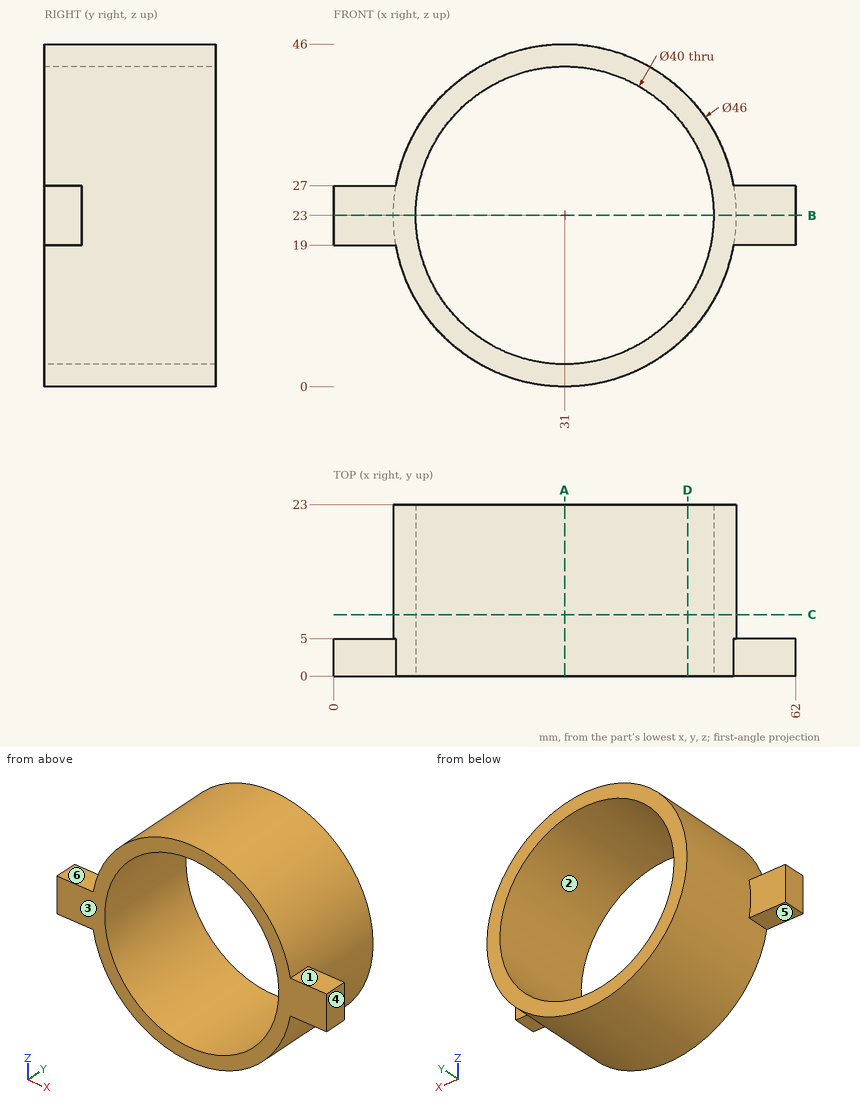
Job drawing, mm, ordinate dimensions from the low corner. One solid piece. A direction names the side the tool comes from. Give positions to 0.01 mm unless a question says otherwise; leave off trailing zeros. Loops run counter-clockwise (first coordinate to the right, second up) from the corner with the lowest first, then second, coordinate; pieces in that order, holes last. Notation, with made-up numbers: (81.25, 24.25) -> (138.25, 24.25) arc R13 ccw to (138.25, 39.25) -> close; hole circle Ø11 at (-16.75, -20.5). An arc over 180 degrees is marked (long way). Use a Markdown table: item, result. Add a question column.
(1) Slice it at C-C on y = 8.25. List the corners of the cut face in (x, z), and give its area (3 significant figures).
(2) Mould opens along Z. For the marked faces 1, 2 and 3 say: +Z half, -Z half, draft (parallel to the pull), parting line (faces both ways), or undercut.
(3) Slice it at B-B on z = 23. List the corners of the cut face in (x, y).
(4) Wall check: line 1 along X through (y, z) = (17, 23); line 2 along Y through (x, z) = (6, 20); line 3 along Z through (x, y) = (46, 14). Give the ranges that are in metal, low to high.
(5) Slice it at D-D on x = 47.5. List the corners of the cut face in (y, z), and give its area (3 significant figures).
(6) Tool access for the marked faces 4, 5 and 6: list every direction of +Z, -Z, +X, -X, +Y, -Y with a clear straight run to the whole face (end or side of a thin tool).
(7) Slice it at A-A on x = 31. List the corners of the cut face in (y, z), and give its area (3 significant figures).
(8) Drop flat-ended pins along their axis: pin 1 Ø4 at (y, z) = (20, 38) entering from -X; pin 2 Ø9 at (x, z) = (59, 24) entering from +Y; pin 3 Ø1.5 at (x, y) = (15, 6.5) entering from +Z. Give the stop position or say it passes through.
Filled sheet:
| question | item | result |
|---|---|---|
| 1 | outline | circle Ø46 at (31, 23); hole circle Ø40 at (31, 23) |
| 1 | area | 405 mm2 |
| 2 | face 1 | +Z half |
| 2 | face 2 | undercut |
| 2 | face 3 | draft |
| 3 | outline | (0, 0) -> (11, 0) -> (11, 23) -> (8, 23) -> (8, 5) -> (0, 5) -> close; (51, 0) -> (62, 0) -> (62, 5) -> (54, 5) -> (54, 23) -> (51, 23) -> close |
| 4 | line 1 | 8 to 11, 51 to 54 |
| 4 | line 2 | 0 to 5 |
| 4 | line 3 | 5.56 to 9.77, 36.23 to 40.44 |
| 5 | outline | (0, 6.98) -> (23, 6.98) -> (23, 11.7) -> (0, 11.7) -> close; (0, 34.3) -> (23, 34.3) -> (23, 39.02) -> (0, 39.02) -> close |
| 5 | area | 217 mm2 |
| 6 | face 4 | +Z, -Z, +X, +Y, -Y |
| 6 | face 5 | -Z, -X, +Y, -Y |
| 6 | face 6 | +Z, -X, +Y, -Y |
| 7 | outline | (0, 0) -> (23, 0) -> (23, 3) -> (0, 3) -> close; (0, 43) -> (23, 43) -> (23, 46) -> (0, 46) -> close |
| 7 | area | 138 mm2 |
| 8 | pin 1 | x = 12.03 |
| 8 | pin 2 | y = 5 |
| 8 | pin 3 | z = 40.22 |
